Geometry check sheet. Reference: the model listing, model coordinates, mm. A direction names the side the tool comes from. Coordinates: 2 decimals unless noted, no trailing zeros. Write each loop counter-clockwise with the first axis right and the second up, starting at its lowest first coordinate (ties: lowest second). Pieces come first, ordered by that corner, then holes. Notation, with made-up numbers: (-0.5, 15) -> (12.5, 15) arc R18 cw to (12.5, 32) -> close; hole circle Ø5 at (6, 63). An arc over 180 degrees is marked (long way). Answer as CSV lines item,"result".
```python
from build123d import *

# Parameters (mm, degrees)
F1_DEPTH = 1
F3_DEPTH = 9
F4_W     = 72
F4_H     = 7
F5_DEPTH = 15
F6_W     = 14
F6_H     = 5
F7_DEPTH = 3


with BuildPart() as f1:
    # F0 (on Front) → F1 (new body)
    with BuildSketch(Plane.XZ):
        with BuildLine():
            ThreePointArc((-10.0408443114, 15.1095405693), (-12.4884072009, 12.922316679), (-13.9832575854, 10))
            Line((-13.9832575854, 10), (-7.5, 10))
            Line((-7.5, 10), (18.5986325968, 10))
            add(Edge.make_bspline(
                [(18.5986325968, 10), (21.7874042537, 17.6571019048), (19.80032664, 26.2314829268)],
                knots=[4.1400176542, 4.1400176542, 4.1400176542, 5.0566635569, 5.0566635569, 5.0566635569], degree=2, weights=[1, 0.8967957597, 1]))
            add(Edge.make_bspline(
                [(12.9993207665, 47.0798322294), (15.450324346, 43.741998707), (20.1470988099, 37.5454970427), (19.5750997548, 26.5514442031), (19.804460929, 26.2712905063), (19.80032664, 26.2314829268)],
                knots=[0, 0, 0, 0, 0.5016072838, 0.9372111202, 1, 1, 1, 1], degree=3))
            ThreePointArc((12.9993207665, 47.0798322294), (15.5438900017, 53.6856045082), (19.5497050621, 47.8491239167))
            ThreePointArc((19.5497050621, 47.8491239167), (19.9685720284, 46.4983646989), (21.3193312462, 46.9172316652))
            ThreePointArc((21.3193312462, 46.9172316652), (16.1624355435, 55.7109825264), (10.5667996719, 47.1896864578))
            add(Edge.make_bspline(
                [(10.5667996719, 47.1896864578), (10.8605309783, 46.7321602294), (11.154313152, 46.2747029689), (11.4453972129, 45.8192883847)],
                knots=[0, 0, 0, 0, 0.0776469035, 0.0776469035, 0.0776469035, 0.0776469035], degree=3))
            add(Edge.make_bspline(
                [(11.4453972129, 45.8192883847), (12.767933728, 43.7501183476), (15.1878409182, 39.878150916), (16.9341324434, 35.7137130449), (17.1275061277, 33.6475465249), (17.2028191458, 32.7424766632)],
                knots=[0.0776469035, 0.0776469035, 0.0776469035, 0.0776469035, 0.430434565, 0.7515396694, 1, 1, 1, 1], degree=3))
            add(Edge.make_bspline(
                [(17.2028191458, 32.7424766632), (14.9801521234, 36.3481891595), (11.8867786303, 37.7342081157)],
                knots=[5.474108615, 5.474108615, 5.474108615, 6.0012992542, 6.0012992542, 6.0012992542], degree=2, weights=[1, 0.9654594475, 1]))
            add(Edge.make_bspline(
                [(11.8867786303, 37.7342081157), (10.7035302137, 45.0083914749), (7.68767306, 49.7129077432)],
                knots=[1.8853250248, 1.8853250248, 1.8853250248, 2.4791891292, 2.4791891292, 2.4791891292], degree=2, weights=[1, 0.9562386323, 1]))
            add(Edge.make_bspline(
                [(7.68767306, 49.7129077432), (6.5442123198, 51.4971863092), (4.4054650757, 54.7938829615), (4.3260539824, 57.9122155888), (4.2892550944, 59.3554241747)],
                knots=[0, 0, 0, 0, 0.5391239155, 1, 1, 1, 1], degree=3))
            Line((4.2892550944, 59.3554241747), (4.2892550944, 62.7361203619))
            add(Edge.make_bspline(
                [(4.2892550944, 62.7361203619), (25.1855731849, 76.6200768708), (3.7327027616, 80.6413343112)],
                knots=[1.8494400705, 1.8494400705, 1.8494400705, 3.9321155412, 3.9321155412, 3.9321155412], degree=2, weights=[1, 0.505066136, 1]))
            Line((3.7327027616, 80.6413343112), (0, 87.0222076774))
            Line((0, 87.0222076774), (-1.7229665969, 80.7154094089))
            add(Edge.make_bspline(
                [(-1.7229665969, 80.7154094089), (-7.5136196625, 79.9089208722), (-12.0973469547, 76.3038908078)],
                knots=[4.3332693398, 4.3332693398, 4.3332693398, 5.1037535185, 5.1037535185, 5.1037535185], degree=2, weights=[1, 0.9267074866, 1]))
            Line((-12.0973469547, 76.3038908078), (-17.5828682239, 79.9423769641))
            Line((-17.5828682239, 79.9423769641), (-16.4939268376, 71.1509964352))
            add(Edge.make_bspline(
                [(-16.4939268376, 71.1509964352), (-24.166699821, 56.1098731464), (-4.2892550944, 59.3554241747)],
                knots=[5.6147383929, 5.6147383929, 5.6147383929, 7.5075967098, 7.5075967098, 7.5075967098], degree=2, weights=[1, 0.5845839527, 1]))
            add(Edge.make_bspline(
                [(-7.68767306, 49.7129077432), (-6.5442123198, 51.4971863092), (-4.4054650757, 54.7938829615), (-4.3260539824, 57.9122155888), (-4.2892550944, 59.3554241747)],
                knots=[0, 0, 0, 0, 0.5391239155, 1, 1, 1, 1], degree=3))
            add(Edge.make_bspline(
                [(-7.68767306, 49.7129077432), (-17.3068218361, 34.7077401912), (-10.0408443114, 15.1095405693)],
                knots=[3.803996178, 3.803996178, 3.803996178, 5.3504242368, 5.3504242368, 5.3504242368], degree=2, weights=[1, 0.7156695663, 1]))
        make_face()
    extrude(amount=F1_DEPTH)

    # F2 (on face) → F3 (join)
    with BuildSketch(Plane.XZ.offset(1)):
        Polygon((-37, 10), (-37, 0), (37, 0), (37, 10), (18.5986325968, 10), (-13.9832575854, 10), align=None)
    extrude(amount=-F3_DEPTH)

    # F4 (on face) → F5 (cut)
    with BuildSketch(Plane(origin=(0, 0, 0), x_dir=(1, 0, 0), z_dir=(0, 0, -1))):
        with Locations((0, -3.5)):
            Rectangle(F4_W, F4_H)
    extrude(amount=-F5_DEPTH, mode=Mode.SUBTRACT)

    # F6 (on face) → F7 (cut)
    with BuildSketch(Plane(origin=(0, 8, 0), x_dir=(-1, 0, 0), z_dir=(0, 1, 0))):
        with Locations((0, 2.5)):
            Rectangle(F6_W, F6_H)
    extrude(amount=-F7_DEPTH, mode=Mode.SUBTRACT)


solid = f1.part
```
Item 1: Cross-section at A-A, the plane x = -31.5. Record the cut outline in (y, z), plus the area to 3 significant figures.
Responses:
outline,"(-1, 0) -> (0, 0) -> (0, 10) -> (-1, 10) -> close; (7, 0) -> (8, 0) -> (8, 10) -> (7, 10) -> close"
area,"20.0 mm2"
Item 2: Set-up check for faces 1 (the flat face through (-14.802, -0.493, 78.098)), 2 (the flat face through (36, 4, 5)), 3 (the flat face through (-1, -1, 34)), 4 (the flat face through (-0.85, -0.49, 83.91)), 5 (the cylindrical face through (-12.46, -0.49, 12.96)): record each of +Z, -Z, +X, -X, +Y, -Y from which the full face is reachable in a straight line by a thin tool's end or side.
Responses:
face 1,"+Z, +Y, -Y"
face 2,"+Z, -Z"
face 3,"+Z, -Z, +X, -X, -Y"
face 4,"+Z, -X, +Y, -Y"
face 5,"-X, +Y, -Y"
Item 3: Release check for a two-part mould opening along Z. For faces 6 (the flat face through (-37, 3, 5)), 7 (the cylindrical face through (16.333, -0.493, 55.704)), 8 (the flat face through (1.89, -0.49, 83.79)) record: +Z half, -Z half, draft (parallel to the pull), parting line (faces both ways), or undercut.
Responses:
face 6,"draft"
face 7,"undercut"
face 8,"+Z half"
Item 4: Thickness scan on probe 1 along Y at (x, z) = (-10.5, 4.5); probe 2 along Y at (x, z) = (-2, 34.5). Record the ranges inside material, lowest first.
Responses:
probe 1,"y = -1 to 0, 7 to 8"
probe 2,"y = -1 to 0"
Item 5: Cross-section at B-B, the plane y = 6. Record the cut outline in (x, z).
Responses:
outline,"(-37, 0) -> (-36, 0) -> (-36, 10) -> (-37, 10) -> close; (36, 0) -> (37, 0) -> (37, 10) -> (36, 10) -> close"
Item 6: Cross-section at C-C, the plane z = 52. Count the separate pieces of the cut face and the enclosed holes in it, plus the area to 3 significant figures.
Responses:
separate pieces,"3"
enclosed holes,"0"
area,"17.1 mm2"
Item 7: Depth check by flat-ended pin: pin 1 Ø21.5 at (x, z) = (6.5, 47) entering from +Y; pin 2 Ø1.1 at (x, y) = (0.5, 7.5) entering from -Z; pin 3 Ø1.1 at (y, z) = (-0.5, 60.5) entering from +X. Enter the tip coordinate at first touch or a pass-through.
Responses:
pin 1,"stops at y = 0"
pin 2,"stops at z = 5"
pin 3,"stops at x = 4.29"
